Work out the finished part from the listing and answer in its coordinate system (mm). Give positions to 0.01 mm unless a question says otherwise; leave off trailing zeros. Write each loop counter-clockwise with the first axis right and the second up, starting at its lowest first coordinate (ties: lowest second). Pieces come first, ordered by that corner, then holes. Notation, with made-up numbers: (0, 51) -> (13, 51) arc R23 ccw to (13, 90) -> close; hole circle Ø10 at (-23.75, 16.5). An arc over 180 degrees is marked (long way). Use a Markdown table: item, result. Add a question column.
Q1. Section A-A, the plane x = 4 is taken. Give the vertices of the cut face in (y, z).
Q2. Section C-C, the plane x = 12.5 is taken. Give the vertices of the cut face in (y, z).
Q3. Consider line 1 (X direction, y = 4, z = 4.5); line 2 (Y direction, x = 21, z = 3.25); line 3 (X direction, y = 3, z = 5.75). Determine where each line is inside the solid, lowest interval first.
Q4. For a pull along Y with two mould halves and no side action, classify faces 1 (the face through (25, 4, 4)), 2 (the face through (0.86, 7.1, 4.06)), 3 (the face through (4.6, 2.847, 3.944)) as pulls with the +Y half, pulls with the -Y half, needs draft (parallel to the pull), parting line crosses it, or undercut.
Q5. Section B-B, the plane z = 4.75 is taken. Give the vertices of the cut face in (x, y).
Q6. This flat-tipped pin is pushed along its axis until it touches: pin 1 Ø1.6 at (x, y) = (4, 4) entering from +Z. Where does it stop, or does it pass through?
Q7. Section D-D, the plane y = 4 is taken. State how many separate pieces and enclosed holes the cut face has, plus the area to 3 significant figures.
from build123d import *

# Parameters (mm, degrees)
CYLINDER002_R     = 3
CYLINDER002_DEPTH = 10
CYLINDER001_R     = 1.3
CYLINDER001_DEPTH = 10
CYLINDER_R        = 1.3
CYLINDER_DEPTH    = 10
BOX_W             = 25
BOX_H             = 8
BOX_DEPTH         = 8
FILLET_R          = 3
FILLET001_R       = 3


with BuildPart() as cylinder002:
    # Cylinder002 → Cylinder002 (new body)
    with BuildSketch(Plane(origin=(12.5, 8, -1), x_dir=(1, 0, 0), z_dir=(0, 0, 1))):
        Circle(CYLINDER002_R)
    extrude(amount=CYLINDER002_DEPTH)


with BuildPart() as cylinder001:
    # Cylinder001 → Cylinder001 (new body)
    with BuildSketch(Plane(origin=(21, 4, -1), x_dir=(1, 0, 0), z_dir=(0, 0, 1))):
        Circle(CYLINDER001_R)
    extrude(amount=CYLINDER001_DEPTH)


with BuildPart() as fusion:
    # Cylinder → Cylinder (new body)
    with BuildSketch(Plane(origin=(4, 4, -1), x_dir=(1, 0, 0), z_dir=(0, 0, 1))):
        Circle(CYLINDER_R)
    extrude(amount=CYLINDER_DEPTH)

    # Fusion: union Cylinder001
    add(cylinder001.part)


with BuildPart() as fillet001:
    # Box → Box (new body)
    with BuildSketch(Plane.XY):
        with Locations((12.5, 4)):
            Rectangle(BOX_W, BOX_H)
    extrude(amount=BOX_DEPTH)

    # Cut: cut Fusion
    add(fusion.part, mode=Mode.SUBTRACT)

    # Fillet
    fillet_edges = [fillet001.edges().sort_by_distance(p)[0] for p in [
        (0, 0, 4),
        (0, 8, 4),
        (25, 0, 4),
        (25, 8, 4),
    ]]
    fillet(fillet_edges, radius=FILLET_R)

    # Cut001: cut Cylinder002
    add(cylinder002.part, mode=Mode.SUBTRACT)

    # Fillet001
    fillet001_edges = [fillet001.edges().sort_by_distance(p)[0] for p in [
        (12.5, 5, 0),
    ]]
    fillet(fillet001_edges, radius=FILLET001_R)


solid = fillet001.part
Result set:
| question | item | result |
|---|---|---|
| 1 | outline | (0, 0) -> (2.7, 0) -> (2.7, 8) -> (0, 8) -> close; (5.3, 0) -> (8, 0) -> (8, 8) -> (5.3, 8) -> close |
| 2 | outline | (0, 0) -> (2, 0) arc R3 ccw to (5, 3) -> (5, 8) -> (0, 8) -> close |
| 3 | line 1 | x = 0 to 2.7, 5.3 to 19.7, 22.3 to 25 |
| 3 | line 2 | y = 0 to 2.7, 5.3 to 8 |
| 3 | line 3 | x = 0 to 3.17, 4.83 to 20.17, 21.83 to 25 |
| 4 | face 1 | needs draft |
| 4 | face 2 | pulls with the +Y half |
| 4 | face 3 | undercut |
| 5 | outline | (0, 3) arc R3 ccw to (3, 0) -> (22, 0) arc R3 ccw to (25, 3) -> (25, 5) arc R3 ccw to (22, 8) -> (15.5, 8) arc R3 cw to (9.5, 8) -> (3, 8) arc R3 ccw to (0, 5) -> close; hole circle Ø2.6 at (4, 4); hole circle Ø2.6 at (21, 4) |
| 6 | pin 1 | passes through |
| 7 | separate pieces | 3 |
| 7 | enclosed holes | 0 |
| 7 | area | 155 mm2 |
